Geometry: final body of the model. Coordinates: model frame, mm. Face numbers are marked on the shaded views. Give positions to 0.01 mm unless a question says otherwise; leave off trailing zeros. Write each loop counter-clockwise with the first axis right and the second up, starting at its lowest first coordinate (ties: lowest second). Pieces come first, ordered by that corner, then holes. Notation, with made-up numbers: (-29.75, 12.25) -> (5.25, 12.25) arc R24 ccw to (5.25, 43.25) -> close; hole circle Ø5 at (87.5, -15.75). An arc over 180 degrees is marked (long way). Use CSV: the item, a comma, the result in double quotes. Start each with the question number.
1) Material intervals for line 1 (X direction, y = -0.25, z = 3); line 2 (Z direction, x = -32, y = 0); line 3 (Y direction, x = -11, z = 0.5), sorted ascending. Write a range as [from, to].
2) Contact query for flat-ended pins moving along their axis: P1, Ø0.8, axis at x = -17, z = 0.5, coming from the +Y side; P2, Ø6, axis at x = -30.5, y = 0.5, coming from the +Z side; P3, Ø1.5, axis at y = 1.5, z = 1, coming from the -X side. Output: stop coordinate, or through.
3) Section A-A (x = 0). Output: boundary loops of the cut face in (y, z) (3 decimals), plus the area to 3 significant figures.
4) Section C-C (y = 6). Output: boundary loops of the cut face in (x, z), plus the area to 3 significant figures.
5) Section D-D (x = 18). Output: boundary loops of the cut face in (y, z).
6) Section B-B (z = 5.25). Output: boundary loops of the cut face in (x, y) (3 decimals), plus the area to 3 significant figures.
7) Draft query along Z for the marked faces 1 and 2. Return one class per face: pulls with the +Z half, pulls with the -Z half, needs draft (parallel to the pull), parting line crosses it, or undercut.
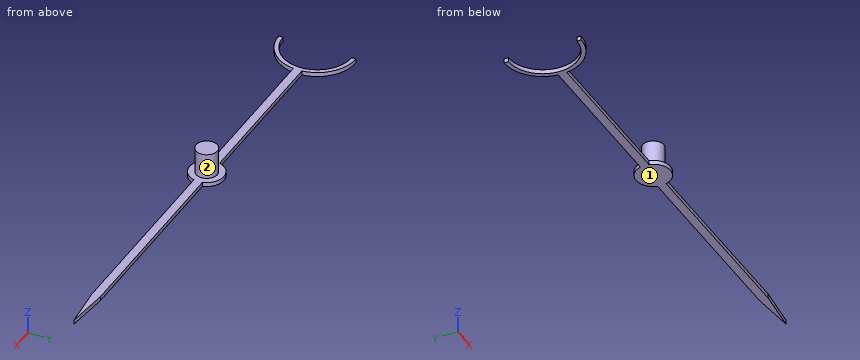
Autodesk Fusion 360 part; units mm, degrees
sketch "Sketch1" plane through (0, 0, 0) normal (0, 0, 1) x (1, 0, 0)
  line L0 (-50, 1) -> (50, -1) construction
  line L1 (50, 1) -> (-50, -1) construction
  line L2 (50, 1) -> (60, 1) construction
  line L3 (50, -1) -> (60, -1) construction
  arc A0 (-50, -8) -> (-50, 8) centre (-50, 0) ccw
  line L4 (-50, 9) -> (-50, 8)
  line L5 (-50, -8) -> (-50, -9)
  line L6 (50, 1) -> (59.9497, -0.002)
  line L7 (59.9497, -0.002) -> (50, -1)
  arc A1 (3.9992, -0.08) -> (3.9992, 0.08) centre (0, 0) ccw
  arc A2 (3.873, 1) -> (-3.873, 1) centre (0, 0) ccw
  arc A3 (-3.9992, 0.08) -> (-3.9992, -0.08) centre (0, 0) ccw
  arc A4 (-3.873, -1) -> (3.873, -1) centre (0, 0) ccw
  arc A5 (-50, -9) -> (-41.0557, -1) centre (-50, 0) ccw
  arc A6 (-41.0557, 1) -> (-50, 9) centre (-50, 0) ccw
  line L8 (-41.0557, 1) -> (-3.873, 1)
  line L9 (3.873, 1) -> (50, 1)
  line L10 (50, -1) -> (3.873, -1)
  line L11 (-3.873, -1) -> (-41.0557, -1)
  dimension "d57" = 8
  dimension "d58" = 100
  dimension "d59" = 2
  dimension "d64" = 8
  dimension "d66" = 10
extrude "Extrude1" add sketch "Sketch1" along normal blind 1
sketch "Sketch2" plane through (0, 0, 1) normal (0, 0, 1) x (-1, 0, 0)
  arc A0 (-3.873, -1) -> (3.873, -1) centre (0, 0) ccw
  line L0 (3.873, -1) -> (41.0557, -1)
  arc A1 (41.0557, -1) -> (50, -9) centre (50, 0) ccw
  line L1 (50, -9) -> (50, -8)
  arc A2 (50, 8) -> (50, -8) centre (50, 0) ccw
  line L2 (50, 8) -> (50, 9)
  arc A3 (50, 9) -> (41.0557, 1) centre (50, 0) ccw
  line L3 (41.0557, 1) -> (3.873, 1)
  arc A4 (3.873, 1) -> (-3.873, 1) centre (0, 0) ccw
  line L4 (-3.873, 1) -> (-50, 1)
  line L5 (-50, 1) -> (-59.9497, 0.002)
  line L6 (-59.9497, 0.002) -> (-50, -1)
  line L7 (-50, -1) -> (-3.873, -1)
  circle A5 centre (0, 0) radius 2.485
  dimension "d69" = 4.97
extrude "Extrude2" add sketch "Sketch2" along normal blind 6 contours A5
Answers follow:
1,line 1,"x = [-2.47, 2.47]"
1,line 2,"z = [0, 1]"
1,line 3,"y = [-1, 1]"
2,P1,"stops at y = 1"
2,P2,"stops at z = 1"
2,P3,"stops at x = -42.32"
3,outline,"(-4, 0) -> (4, 0) -> (4, 1) -> (2.485, 1) -> (2.485, 7) -> (-2.485, 7) -> (-2.485, 1) -> (-4, 1) -> close"
3,area,"37.8 mm^2"
4,outline,"(-44.71, 0) -> (-43.29, 0) -> (-43.29, 1) -> (-44.71, 1) -> close"
4,area,"1.42 mm^2"
5,outline,"(-1, 0) -> (1, 0) -> (1, 1) -> (-1, 1) -> close"
6,outline,"circle Ø4.97 at (0, 0)"
6,area,"19.4 mm^2"
7,face 1,"pulls with the -Z half"
7,face 2,"needs draft"
